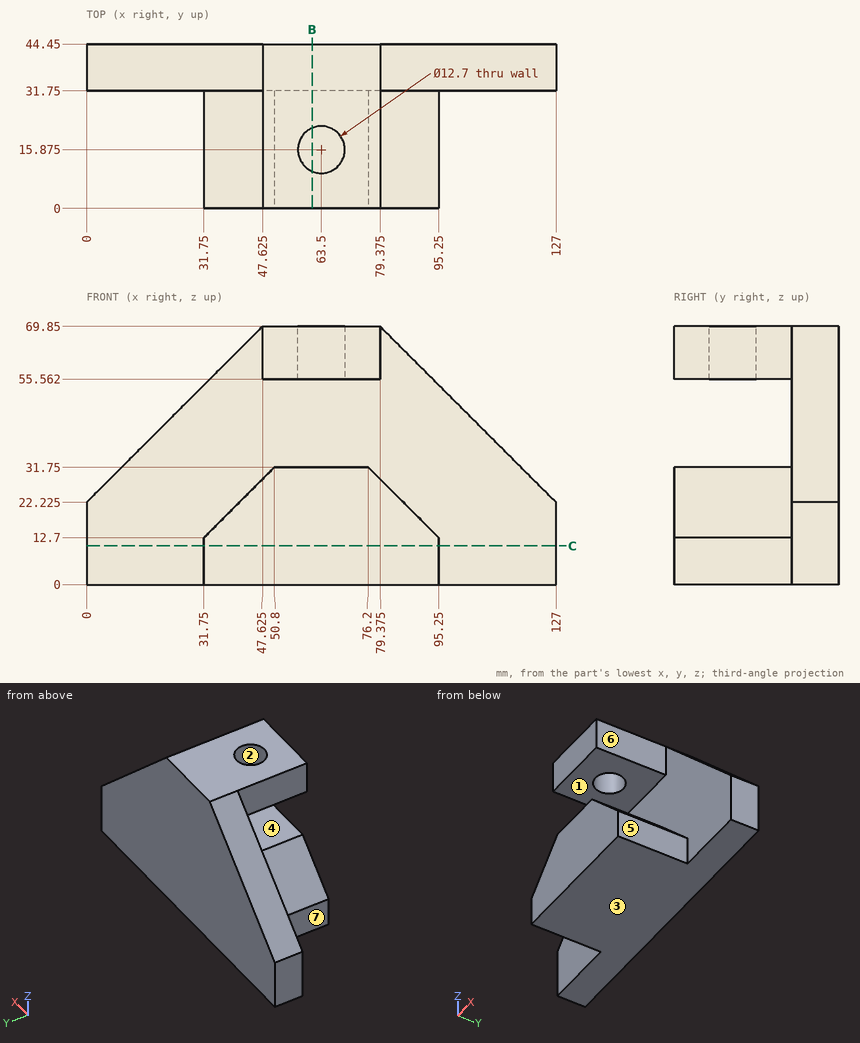
Verification items for this drawing (mm, ordinates from the low corner). A direction names the side the tool comes from. Coordinates: 2 decimals unless noted, no trailing zeros. Order: outer loops, then holes, each group sorted by start corner. A loop starts at its lowest first (then second) coordinate and runs counter-clockwise, first axis right, second up.
Q1. Sectioned sample at B-B on x = 61. Record the cut outline in (y, z), and give its area (3 significant figures).
Reply:
outline: (0, 0) - (44.45, 0) - (44.45, 69.85) - (21.71, 69.85) - (21.71, 55.56) - (31.75, 55.56) - (31.75, 31.75) - (0, 31.75) - close; (0, 55.56) - (10.04, 55.56) - (10.04, 69.85) - (0, 69.85) - close
area: 2,180 mm2
Q2. Thickness scan on probe 1 along Z at (x, y) = (60.5, 6.5); probe 2 along X at (y, z) = (7, 8); probe 3 along Y at (x, z) = (95.5, 22). Record the ranges inside material, lowest first.
Reply:
probe 1: z = 0 to 31.75, 55.56 to 69.85
probe 2: x = 31.75 to 95.25
probe 3: y = 31.75 to 44.45
Q3. Draft check along Z on the marked faces 1, 2 and 3. Enter one of: released by +Z, released by -Z, zero draft, split by the parting line, or undercut.
Reply:
face 1: undercut
face 2: zero draft
face 3: released by -Z
Q4. Depth check by flat-ended pin: pin 1 Ø4 at (y, z) = (16.5, 3.5) entering from +X; pin 2 Ø10 at (y, z) = (8.5, 4.5) entering from -X; pin 3 Ø2 at (x, z) = (53, 42) entering from -Y. Enter the tip coordinate at first touch or a pass-through.
Reply:
pin 1: stops at x = 95.25
pin 2: stops at x = 31.75
pin 3: stops at y = 31.75
Q5. Sectioned sample at C-C on z = 10.5. Record the cut outline in (x, y), and give its area (3 significant figures).
Reply:
outline: (0, 31.75) - (31.75, 31.75) - (31.75, 0) - (95.25, 0) - (95.25, 31.75) - (127, 31.75) - (127, 44.45) - (0, 44.45) - close
area: 3,630 mm2
Q6. Tool access check on the marked faces 4, 5, 6 and 7. Record the directions out of +Z, -Z, +X, -X, +Y, -Y that give a thin tool (end or side, any length) a straight path to the whole face; none if there is none.
Reply:
face 4: +X, -X, -Y
face 5: +Z, -Z, +X, -Y
face 6: +Z, +X, -Y
face 7: +Z, -Z, -X, -Y
